Check sheet for the modelled part. Datum: model origin and axes. Units: mm. Face numbers are marked on the shaded views. Round coordinates to 2 decimals unless told otherwise and drop trailing zeros. Loops run counter-clockwise (first coordinate to the right, second up) from the corner with the lowest first, then second, coordinate; pieces in that order, holes last. Notation, with made-up numbers: (-40, 30) -> (-34, 30) arc R17 cw to (-34, 51) -> close; hole circle Ø5 at (-11.75, 67). An arc over 180 degrees is marked (long way). One line per item, written item: value. Start each with the question number.
1. Release check for a two-part mould opening along Y. For the marked faces 1, 2 and 3 record: +Y half, -Y half, draft (parallel to the pull), parting line (faces both ways), or undercut.
2. Material ranges on L1, parallel to Y at x = -2, z = 0.5; L2, parallel to X at y = -3.2, z = -0.25; L3, parallel to Y at x = 1, z = 2.25, recorded low to high.
3. Go/stop test with flat-tipped pins: pin 1 (2 mm diameter, centred on y = 0, z = 2, fed in from -X); pin 2 (1 mm diameter, centred on x = 1.5, y = -2.5, fed in from +Z); pin 3 (2 mm diameter, centred on x = 0.5, z = -0.5, fed in from -Y); pin 4 (3 mm diameter, centred on x = 0, z = 0.5, fed in from +Y). Record where each tip stops, or that it passes through.
4. Cross-section at C-C on y = -0.2. Record the cut outline in (x, z).
from build123d import *


with BuildPart() as part:
    # Sketch1 → Revolve1 (revolve)
    with BuildSketch(Plane.XY):
        with BuildLine():
            Line((4, 0.129563319), (4, 0.1))
            ThreePointArc((4, 0.1), (3.970710678, 0.029289322), (3.9, 0))
            Line((3.9, 0), (2, 0))
            Line((2, 0), (2, -2.4))
            Line((2, -2.4), (2.5, -2.4))
            ThreePointArc((2.5, -2.4), (3, -2.9), (2.5, -3.4))
            Line((2.5, -3.4), (1.9, -3.4))
            ThreePointArc((1.9, -3.4), (1.546446609, -3.253553391), (1.4, -2.9))
            Line((1.4, -2.9), (0, -2.9))
            Line((0, -2.9), (0, 0.9))
            ThreePointArc((0, 0.9), (1.99554555, 0.729724866), (3.933394495, 0.223822576))
            ThreePointArc((3.933394495, 0.223822576), (3.981668383, 0.187271856), (4, 0.129563319))
        make_face()
    revolve(axis=Axis((0, 0, 0), (0, -1, 0)))


solid = part.part
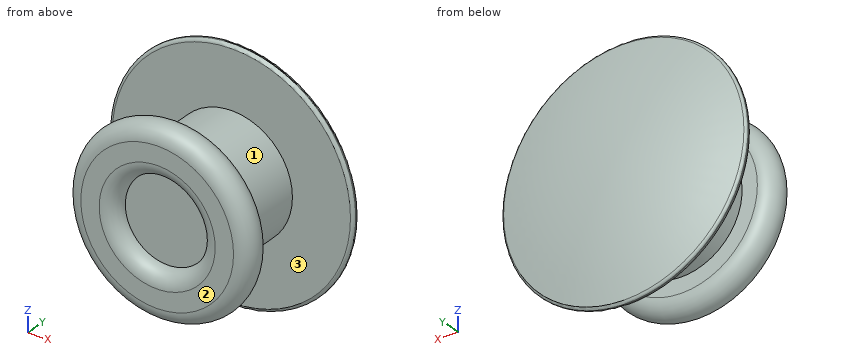
Taken from the geometry:
1. face 1: undercut
1. face 2: -Y half
1. face 3: undercut
2. L1: y = -3.4 to -2.4, 0 to 0.72
2. L2: x = -2.89 to -1.48, 1.48 to 2.89
2. L3: y = -3.4 to -2.4, 0 to 0.64
3. pin 1: stops at x = -3.87
3. pin 2: stops at z = 2.78
3. pin 3: stops at y = -3.36
3. pin 4: stops at y = 0.9
4. outline: circle Ø4 at (0, 0)
